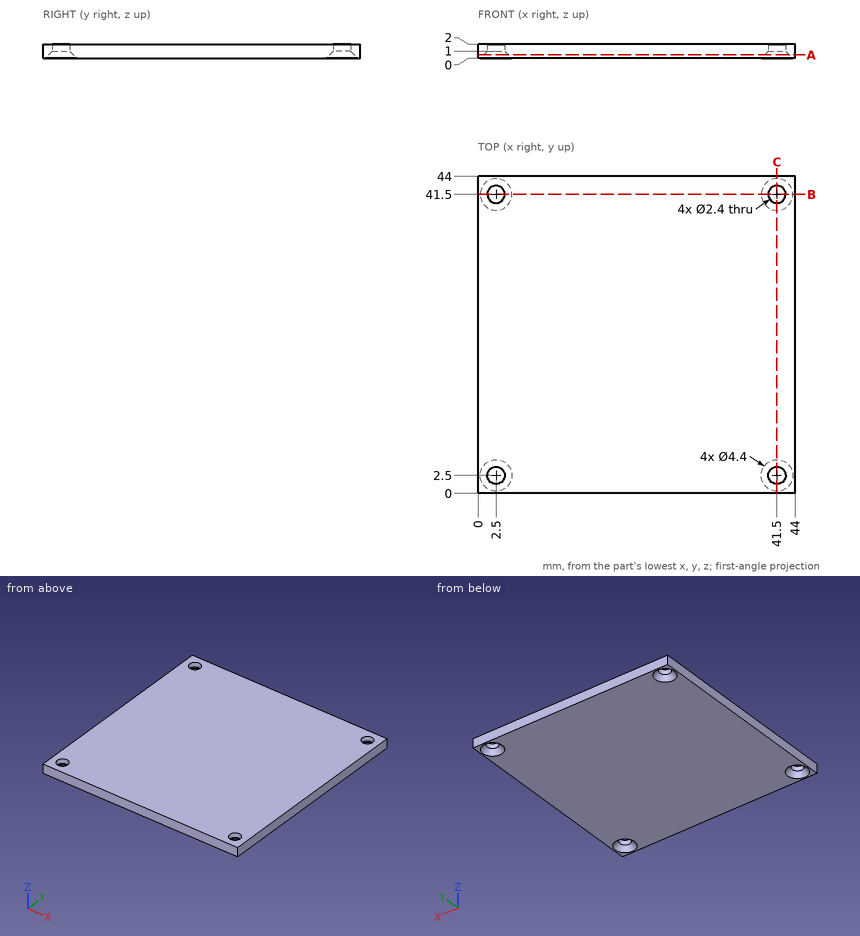
Check sheet for the drawn part. Datum: minimum x, y, z corner. Units: mm. Coordinates: 2 decimals unless noted, no trailing zeros. Write each loop counter-clockwise with the first axis right and the second up, starting at its lowest first coordinate (ties: lowest second). Pieces come first, ordered by that corner, then holes. Notation, with made-up numbers: M -38,33.25 L -4,33.25 A34 cw -4,70.25 Z; hole C 85.5,21.25 d2. An arc over 180 degrees is marked long. Use a Markdown table: item, result.
Q1. Go/stop test with a flat-tipped pin: P1, Ø3, axis at x = 2.5, y = 2.5, coming from the -Z side. Record where the tip stops, or that it passes through.
Reply:
| item | result |
|---|---|
| P1 | stops at z = 0.7 |
Q2. Sectioned sample at B-B, the plane y = 41.5. Record the boundary of the cut face in (x, z), plus the area to 3 significant figures.
Reply:
| item | result |
|---|---|
| outline | M 0,0 L 0.3,0 L 1.3,1 L 1.3,2 L 0,2 Z; M 3.7,1 L 4.7,0 L 39.3,0 L 40.3,1 L 40.3,2 L 3.7,2 Z; M 42.7,1 L 43.7,0 L 44,0 L 44,2 L 42.7,2 Z |
| area | 76.4 mm² |
Q3. Thickness scan on line 1 (X direction, y = 2.5, z = 1.3); line 2 (Y direction, x = 40.5, z = 1.6). Record the ranges inside material, lowest first.
Reply:
| item | result |
|---|---|
| line 1 | x = 0 to 1.3, 3.7 to 40.3, 42.7 to 44 |
| line 2 | y = 0 to 1.84, 3.16 to 40.84, 42.16 to 44 |
Q4. Sectioned sample at A-A, the plane z = 0.5. Record the boundary of the cut face in (x, y), plus the area to 3 significant figures.
Reply:
| item | result |
|---|---|
| outline | M 0,0 L 44,0 L 44,44 L 0,44 Z; hole C 2.5,2.5 d3.4; hole C 2.5,41.5 d3.4; hole C 41.5,2.5 d3.4; hole C 41.5,41.5 d3.4 |
| area | 1,900 mm² |
